Here's how the part is built. I have some questions about the finished solid (model axes, mm). Give positions to 0.01 mm unless a question says otherwise; leave off trailing zeros. Loops run counter-clockwise (first coordinate to the right, second up) from the corner with the lowest first, then second, coordinate; pieces in that order, holes last. Notation, with made-up numbers: M 57,41 L 76,41 A17 cw 76,59 Z; hole C 76,36 d9. An arc over 180 degrees is marked long. Write item = value, one per line. Start each with the question number.
```python
from build123d import *

# Parameters (mm, degrees)
F0_W     = 31.75
F0_H     = 11.1125
F1_DEPTH = 25.4
F3_DEPTH = 6.35


with BuildPart() as f1:
    # F0 (on Front) → F1 (new body)
    with BuildSketch(Plane.XZ):
        Rectangle(F0_W, F0_H)
    extrude(amount=F1_DEPTH)

    # F2 (on face) → F3 (cut)
    with BuildSketch(Plane(origin=(-15.875, 0, 0), x_dir=(0, -1, 0), z_dir=(-1, 0, 0))):
        with BuildLine():
            ThreePointArc((12.7, -1.5), (13.76066, -1.06066), (14.2, 0))
            ThreePointArc((14.2, 0), (11.63934, 1.06066), (12.7, -1.5))
        make_face()
    extrude(amount=-F3_DEPTH, mode=Mode.SUBTRACT)


solid = f1.part
```
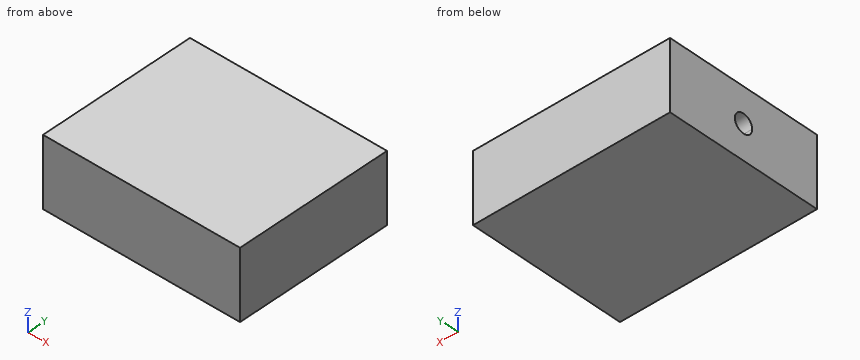
Q1. If we section it at A-A, the plane x = -13.5: List the corners of the cut face in (y, z) for me.
Q2. If I drill on line 1 along Z through (x, y) = (-12.5, -12.7); line 2 along Y through (x, z) = (-13.5, 0), over which ranges is the centre line in solid material (lowest first)?
Q3. If we section it at B-B, the plane z = 1: List the corners of the cut face in (x, y) for me (3 decimals), then the cut area to 3 significant figures.
Q4. Will these pins go through, and if not, where does the flat tip stop? pin 1 (5 mm diameter, centred on x = 8.5, z = -1, fed in from +Y); pin 2 (2.5 mm diameter, centred on y = -12.5, z = 0, fed in from -X) (3 decimals).
Resolved:
q1.outline = M -25.4,-5.56 L 0,-5.56 L 0,5.56 L -25.4,5.56 Z; hole C -12.7,0 d3
q2.line_1 = -5.56 to -1.5, 1.5 to 5.56
q2.line_2 = -25.4 to -14.2, -11.2 to 0
q3.outline = M -15.875,-25.4 L 15.875,-25.4 L 15.875,0 L -15.875,0 L -15.875,-11.582 L -9.525,-11.582 L -9.525,-13.818 L -15.875,-13.818 Z
q3.area = 792 mm²
q4.pin_1 = 0
q4.pin_2 = -9.525
